from build123d import *

# Parameters (mm, degrees)
BOSS_EXTRUDE1_DEPTH = 20
SKETCH3_R           = 6
SKETCH3_R_2         = 2.5
CUT_EXTRUDE1_DEPTH  = 40


with BuildPart() as part:
    # Sketch1 → Boss-Extrude1 (new, symmetric)
    with BuildSketch(Plane.XY):
        with BuildLine():
            Line((0, 2), (0, 50))
            Line((0, 50), (2, 50))
            Line((2, 50), (2, 4))
            ThreePointArc((2, 4), (2.585786438, 2.585786438), (4, 2))
            Line((4, 2), (50, 2))
            Line((50, 2), (50, 0))
            Line((50, 0), (2, 0))
            ThreePointArc((2, 0), (0.585786438, 0.585786438), (0, 2))
        make_face()
    extrude(amount=BOSS_EXTRUDE1_DEPTH, both=True)

    # Sketch3 → Cut-Extrude1 (cut)
    with BuildSketch(Plane(origin=(0, 2, 0), x_dir=(1, 0, 0), z_dir=(0, 1, 0))):
        with Locations(Location((27.405417893, 0, 0), (0, 0, 270))):
            Circle(SKETCH3_R)
        with Locations(Location((40.675078118, 12.5, 0), (0, 0, 270))):
            Circle(SKETCH3_R_2)
        with Locations(Location((40.675078118, -12.5, 0), (0, 0, 270))):
            Circle(SKETCH3_R_2)
        with Locations(Location((14.107643981, -12.5, 0), (0, 0, 270))):
            Circle(SKETCH3_R_2)
        with Locations(Location((14.107643981, 12.5, 0), (0, 0, 270))):
            Circle(SKETCH3_R_2)
    cut_extrude1 = extrude(amount=-CUT_EXTRUDE1_DEPTH, mode=Mode.SUBTRACT)

    # Mirror1: Cut-Extrude1 across plane
    add(cut_extrude1.mirror(Plane(origin=(0, 0, 0), x_dir=(0, 0, 1), z_dir=(-0.7071067811865488, 0.7071067811865464, 0))), mode=Mode.SUBTRACT)


solid = part.part
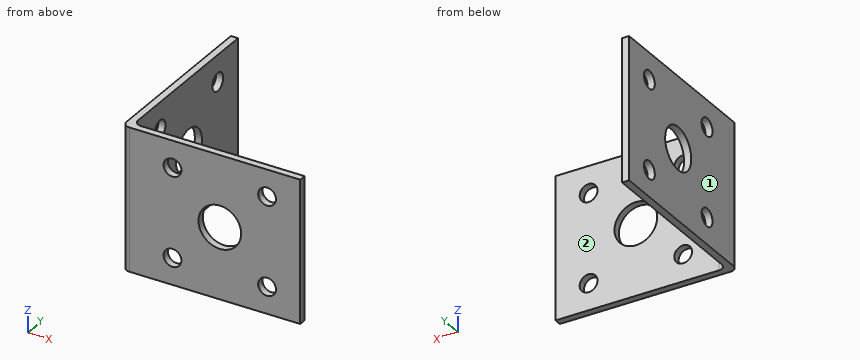
The listing builds one solid part. Answer for the finished solid, in the listing's coordinates (mm). Face numbers are marked on the shaded views. A direction names the side the tool comes from. Coordinates: 2 decimals unless noted, no trailing zeros. Loops run counter-clockwise (first coordinate to the right, second up) from the corner with the lowest first, then second, coordinate; pieces in that order, holes last.
1) Find section C-C on x = 31. Write down the section's boundary in (y, z), then the cut area to 3 significant figures.
2) Flat-ended cylindrical pins translate along their axes: pin 1 Ø8 at (x, z) = (40.68, -12.5) entering from +Y; pin 2 Ø3 at (x, z) = (14.11, 12.5) entering from -Y; pin 3 Ø6 at (x, z) = (14.11, -12.5) entering from -Y; pin 4 Ø8 at (y, z) = (19.5, 15) entering from +X. Find the tip coordinate at first contact, or state that the pin passes through.
3) Find the intervals of material crossed by L1, parallel to Y at x = 1, z = -12; L2, parallel to X at y = 23.5, z = 16.5, in increasing order.
4) A tool of negligible diameter and unlimited length cuts with its end or side. For the marked faces 1 and 2, from which of +Z, -Z, +X, -X, +Y, -Y can it reach the whole face along a straight path? Write none if from no direction.
5) Find section A-A on z = 12.5. Write down the section's boundary in (x, y).
6) Find section D-D on y = 22.5. Write down the section's boundary in (x, z).
7) Find section B-B on z = 0. Write down the section's boundary in (x, y).
Values:
1. outline: (0, -20) - (2, -20) - (2, -4.8) - (0, -4.8) - close; (0, 4.8) - (2, 4.8) - (2, 20) - (0, 20) - close
1. area: 60.8 mm2
2. pin 1: stops at y = 2
2. pin 2: passes through
2. pin 3: stops at y = 0
2. pin 4: stops at x = 2
3. L1: y = 0.27 to 11.66, 16.56 to 38.23, 43.12 to 50
3. L2: x = 0 to 2
4. face 1: +Z, -Z, -X, +Y, -Y
4. face 2: +Z, -Z, +X, +Y
5. outline: (0, 2) arc R2 ccw to (2, 0) - (11.61, 0) - (11.61, 2) - (4, 2) arc R2 cw to (2, 4) - (2, 11.61) - (0, 11.61) - close; (0, 16.61) - (2, 16.61) - (2, 38.18) - (0, 38.18) - close; (0, 43.18) - (2, 43.18) - (2, 50) - (0, 50) - close; (16.61, 0) - (38.18, 0) - (38.18, 2) - (16.61, 2) - close; (43.18, 0) - (50, 0) - (50, 2) - (43.18, 2) - close
6. outline: (0, -20) - (2, -20) - (2, -3.45) - (0, -3.45) - close; (0, 3.45) - (2, 3.45) - (2, 20) - (0, 20) - close
7. outline: (0, 2) arc R2 ccw to (2, 0) - (21.41, 0) - (21.41, 2) - (4, 2) arc R2 cw to (2, 4) - (2, 21.41) - (0, 21.41) - close; (0, 33.41) - (2, 33.41) - (2, 50) - (0, 50) - close; (33.41, 0) - (50, 0) - (50, 2) - (33.41, 2) - close
